```python
from build123d import *

# Parameters (mm, degrees)
SKETCH_W                = 10
SKETCH_H                = 10
PAD_DEPTH               = 5
SKETCH001_R             = 2
PAD001_DEPTH            = 2
SKETCH002_R             = 1
POCKET_DEPTH            = 38.560468
CHAMFER_SIZE            = 0.6
SKETCH001_MIRRORED_2_R  = 2
PAD001_MIRRORED_2_DEPTH = 2


with BuildPart() as part:
    # Sketch → Pad (new body)
    with BuildSketch(Plane.XY):
        Rectangle(SKETCH_W, SKETCH_H)
    extrude(amount=PAD_DEPTH)

    # Sketch001 (on Face6 of Pad) → Pad001 (join)
    with BuildSketch(Plane.XY.offset(5)):
        with Locations((2.5, 2.5)):
            Circle(SKETCH001_R)
    pad001 = extrude(amount=PAD001_DEPTH)

    # Sketch002 (on Face8 of Pad001) → Pocket (cut, through all)
    with BuildSketch(Plane.XY.offset(7)):
        with Locations((2.5, 2.5)):
            Circle(SKETCH002_R)
    pocket = extrude(amount=-POCKET_DEPTH, mode=Mode.SUBTRACT)

    # Chamfer
    chamfer_edges = [part.edges().sort_by_distance(p)[0] for p in [
        (0.5, 2.5, 7),
    ]]
    chamfer(chamfer_edges, length=CHAMFER_SIZE)

    # Sketch001 Mirrored 2 → Pad001 Mirrored 2 (add)
    with BuildSketch(Plane(origin=(0, 0, 5), x_dir=(-1, 0, 0), z_dir=(0, 0, -1))):
        with Locations((2.5, 2.5)):
            Circle(SKETCH001_MIRRORED_2_R)
    pad001_mirrored_2 = extrude(amount=-PAD001_MIRRORED_2_DEPTH)

    # Mirrored001: Pad001, Pad001 Mirrored 2 across XZ
    add(pad001.mirror(Plane.XZ))
    add(pad001_mirrored_2.mirror(Plane.XZ))

    # Mirrored002: Pocket across Sketch002 V_Axis
    add(pocket.mirror(Plane(origin=(0, 0, 7), x_dir=(0, 0, 1), z_dir=(1, 0, 0))), mode=Mode.SUBTRACT)


solid = part.part
```
Geometry: final body of the model. Coordinates: model frame, mm. A direction names the side the tool comes from. Round coordinates to 2 decimals unless told otherwise and drop trailing zeros. Write each loop counter-clockwise with the first axis right and the second up, starting at its lowest first coordinate (ties: lowest second). Pieces come first, ordered by that corner, then holes.
Item 1: Section query D-D (y = -2.5). Return loops of the section in (x, z), plus the area to 3 significant figures.
Item 2: Material intervals for L1, parallel to Y at x = -2.5, z = 4.75; L2, parallel to Y at x = -3.25, z = 6.75; L3, parallel to Z at x = -0.25, y = -2.25, sorted ascending.
Item 3: Section query A-A (y = 2.5). Return loops of the section in (x, z), plus the area to 3 significant figures.
Item 4: Mould query, pull axis Y, two halves, no side actions, for faces 3 (the face through (-2.066, -0.548, 5.986)), 4 (the face through (0, -5, 2)), 5 (the face through (2, -3, 7)). Classes: +Y half, -Y half, draft (parallel to the pull), parting line (faces both ways), or undercut.
Item 5: Pin query (flat end, axial travel): P1, Ø2.5, axis at x = 2.5, y = 2.5, coming from the +Z side. Return the tip coordinate at first contact, or that it passes through.
Item 6: Set-up query: faces 1 (the face through (0, 5, 2)), 2 (the face through (2.066, -0.548, 5.986)). Return all of +Z, -Z, +X, -X, +Y, -Y with unobstructed straight access to the full face (end or side cutting, diameter ignored); none if empty.
Item 7: Section query C-C (z = 2.75). Return loops of the section in (x, y).
Item 8: Section query B-B (x = 2.5). Return loops of the section in (y, z).
Completed:
1. outline: (-5, 0) - (5, 0) - (5, 5) - (4.5, 5) - (4.5, 7) - (0.5, 7) - (0.5, 5) - (-0.5, 5) - (-0.5, 7) - (-4.5, 7) - (-4.5, 5) - (-5, 5) - close
1. area: 66.0 mm2
2. L1: y = -5 to 1.5, 3.5 to 5
2. L2: y = -4.35 to -0.65, 0.65 to 1.84, 3.16 to 4.35
2. L3: z = 0 to 5
3. outline: (-5, 0) - (-3.5, 0) - (-3.5, 7) - (-4.5, 7) - (-4.5, 5) - (-5, 5) - close; (-1.5, 0) - (1.5, 0) - (1.5, 7) - (1.1, 7) - (0.5, 6.4) - (0.5, 5) - (-0.5, 5) - (-0.5, 7) - (-1.5, 7) - close; (3.5, 0) - (5, 0) - (5, 5) - (4.5, 5) - (4.5, 6.4) - (3.9, 7) - (3.5, 7) - close
3. area: 37.6 mm2
4. face 3: undercut
4. face 4: -Y half
4. face 5: draft
5. P1: stops at z = 7
6. face 1: +Z, -Z, +X, -X, +Y
6. face 2: +Z
7. outline: (-5, -5) - (5, -5) - (5, 5) - (-5, 5) - close; hole circle Ø2 at (-2.5, 2.5); hole circle Ø2 at (2.5, 2.5)
8. outline: (-5, 0) - (1.5, 0) - (1.5, 7) - (1.1, 7) - (0.5, 6.4) - (0.5, 5) - (-0.5, 5) - (-0.5, 7) - (-4.5, 7) - (-4.5, 5) - (-5, 5) - close; (3.5, 0) - (5, 0) - (5, 5) - (4.5, 5) - (4.5, 6.4) - (3.9, 7) - (3.5, 7) - close
